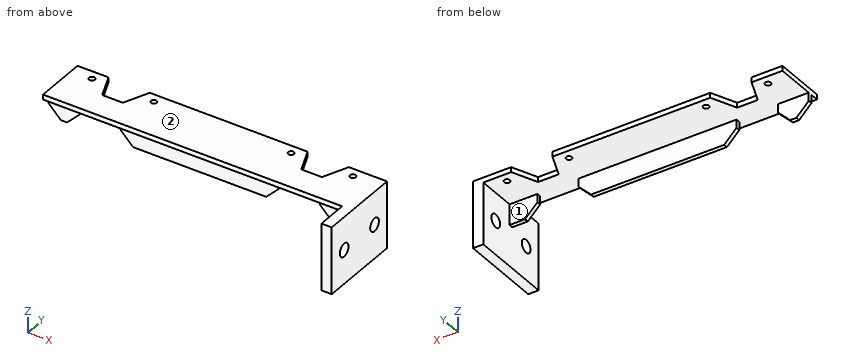
from build123d import *

# Parameters (mm, degrees)
SKETCH1_W                       = 150
SKETCH1_H                       = 25
BOSS_EXTRUDE1_DEPTH             = 2.4
SKETCH2_R                       = 1.4
CUT_EXTRUDE1_DEPTH              = 153.088000842
SKETCH3_W                       = 5
SKETCH3_H                       = 40
BOSS_EXTRUDE2_DEPTH             = 30
BOSS_EXTRUDE2_DIRECTION_2_REACH = 154.088
SKETCH4_R                       = 3.15
CUT_EXTRUDE2_DEPTH              = 30
SKETCH8_W                       = 10
SKETCH8_H                       = 2
BOSS_EXTRUDE4_DEPTH             = 145
SKETCH9_W                       = 20
SKETCH9_H                       = 12.540874848
SKETCH9_H_2                     = 13.006860614
CUT_EXTRUDE4_DEPTH              = 159.113883008
CHAMFER5_SIZE                   = 6


with BuildPart() as part:
    # Sketch1 → Boss-Extrude1 (new body)
    with BuildSketch(Plane.XY):
        with Locations((75, 12.5)):
            Rectangle(SKETCH1_W, SKETCH1_H)
    extrude(amount=BOSS_EXTRUDE1_DEPTH)

    # Sketch2 → Cut-Extrude1 (cut, through all)
    with BuildSketch(Plane.XY.offset(2.4)):
        with Locations((40, 20.5)):
            Circle(SKETCH2_R)
        with Locations(Location((10, 20.5, 0), (0, 0, 180))):
            Circle(SKETCH2_R)
        with Locations(Location((106.5, 20.5, 0), (0, 0, 180))):
            Circle(SKETCH2_R)
        with Locations((136.5, 20.5)):
            Circle(SKETCH2_R)
        Polygon((131.5, 25), (126.5, 13), (116.5, 13), (111.5, 25), align=None)
        Polygon((35, 25), (30, 13), (20, 13), (15, 25), align=None)
    extrude(amount=-CUT_EXTRUDE1_DEPTH, mode=Mode.SUBTRACT)

    # Sketch3 → Boss-Extrude2 (add)
    with BuildSketch(Plane(origin=(0, 0, 0), x_dir=(-1, 0, 0), z_dir=(0, 0, -1))):
        with Locations((-147.5, 5)):
            Rectangle(SKETCH3_W, SKETCH3_H)
    extrude(amount=BOSS_EXTRUDE2_DEPTH)

    # Boss-Extrude2 direction 2: up to this face of the body (flat: up to its plane)
    boss_extrude2_direction_2_end = Plane(part.part.faces().sort_by_distance((75.200008519, 11.67481859, 2.4))[0])
    # Sketch3 → Boss-Extrude2 direction 2 (add, up to the picked face)
    with BuildSketch(Plane(origin=(0, 0, 0), x_dir=(-1, 0, 0), z_dir=(0, 0, -1)), mode=Mode.PRIVATE) as boss_extrude2_direction_2_sk1:
        with Locations((-147.5, 5)):
            Rectangle(SKETCH3_W, SKETCH3_H)
    boss_extrude2_direction_2_tool1 = split(extrude(boss_extrude2_direction_2_sk1.sketch, amount=-BOSS_EXTRUDE2_DIRECTION_2_REACH, mode=Mode.PRIVATE), bisect_by=boss_extrude2_direction_2_end, keep=Keep.BOTH, mode=Mode.PRIVATE)
    add(boss_extrude2_direction_2_tool1.solids().sort_by(Axis((147.5, 5, 0), (0, 0, 1)))[0])

    # Sketch4 → Cut-Extrude2 (cut)
    with BuildSketch(Plane.ZY.offset(-145)):
        with Locations((-13.6, 16)):
            Circle(SKETCH4_R)
        with Locations((-13.6, -6)):
            Circle(SKETCH4_R)
    extrude(amount=-CUT_EXTRUDE2_DEPTH, mode=Mode.SUBTRACT)

    # Sketch8 → Boss-Extrude4 (add)
    with BuildSketch(Plane.ZY.offset(-145)):
        with Locations((-5, 5)):
            Rectangle(SKETCH8_W, SKETCH8_H)
    extrude(amount=BOSS_EXTRUDE4_DEPTH)

    # Sketch9 → Cut-Extrude4 (cut, through all)
    with BuildSketch(Plane(origin=(0, 25, 0), x_dir=(1, 0, 0), z_dir=(0, 1, 0))):
        with Locations((121.5, 6.270437424)):
            Rectangle(SKETCH9_W, SKETCH9_H)
        with Locations((25, 6.503430307)):
            Rectangle(SKETCH9_W, SKETCH9_H_2)
    extrude(amount=-CUT_EXTRUDE4_DEPTH, mode=Mode.SUBTRACT)

    # Chamfer5
    chamfer5_edges = [part.edges().sort_by_distance(p)[0] for p in [
        (111.5, 5, -10),
        (131.5, 5, -10),
        (15, 5, -10),
        (35, 5, -10),
        (0, 5, -10),
    ]]
    chamfer(chamfer5_edges, length=CHAMFER5_SIZE)


solid = part.part
Can you work these out from the model? Positions are in its coordinate system, mm. Face numbers are marked on the shaded views. A direction names the side the tool comes from. Coordinates: 2 decimals unless noted, no trailing zeros. Write each loop counter-clockwise with the first axis right and the second up, starting at its lowest first coordinate (ties: lowest second). Pieces come first, ordered by that corner, then holes. Notation, with made-up numbers: (-20.5, 37.5) -> (-1.5, 37.5) arc R12 cw to (-1.5, 59.5) -> close; hole circle Ø4 at (-15.75, 56.25). An arc over 180 degrees is marked (long way). Write each question's results on one line, items separated by ' | '. Start each with the question number.
Item 1: If we section it at D-D, the plane x = 81: Write out the boundary of the cut face in (y, z), and give its area (3 significant figures).
Item 2: Please list where these lines run through material, in increasing order: probe 1 along Y at (x, z) = (10, 0.95); probe 2 along Y at (x, z) = (148, -13); probe 3 along X at (y, z) = (9.5, -4).
Item 3: I'm going to push flat-ended pins straight in: P1, Ø3, axis at x = 91, z = -5.5, coming from the +Y side; P2, Ø12, axis at x = 56, z = -5, coming from the -Y side; P3, Ø0.7, axis at x = 121, z = 1, coming from the +Y side. Where does each tip first touch, or does it pass through?
Item 4: On a 3-axis mill with a long thin cutter (end or side, diameter ignored), from which of +Z, -Z, +X, -X, +Y, -Y can I reach the whole of each face in a straight line? I mean the marked faces 1 and 2. Say none if no direction works.
Item 5: If we section it at A-A, the plane y = -6: Write out the boundary of the cut face in (x, z).
Item 6: If we section it at B-B, the plane z = -13.6: Write out the boundary of the cut face in (x, y).
Item 7: If we section it at C-C, the plane y = 20.5: Count the separate pieces of the cut face and the enclosed holes in it, and give its area (3 significant figures).
Answer block:
1) outline: (0, 0) -> (4, 0) -> (4, -10) -> (6, -10) -> (6, 0) -> (25, 0) -> (25, 2.4) -> (0, 2.4) -> close | area: 80.0 mm²
2) probe 1: 0 to 19.1, 21.9 to 25 | probe 2: -15 to -9.09, -2.91 to 12.91, 19.09 to 25 | probe 3: 145 to 150
3) P1: y = 6 | P2: y = 0 | P3: y = 13
4) face 1: -Z, -X, +Y | face 2: +Z, +X, -X, +Y, -Y
5) outline: (145, -30) -> (150, -30) -> (150, -16.75) -> (145, -16.75) -> close; (145, -10.45) -> (150, -10.45) -> (150, 2.4) -> (145, 2.4) -> close
6) outline: (145, -15) -> (150, -15) -> (150, -9.15) -> (145, -9.15) -> close; (145, -2.85) -> (150, -2.85) -> (150, 12.85) -> (145, 12.85) -> close; (145, 19.15) -> (150, 19.15) -> (150, 25) -> (145, 25) -> close
7) separate pieces: 7 | enclosed holes: 0 | area: 405 mm²
